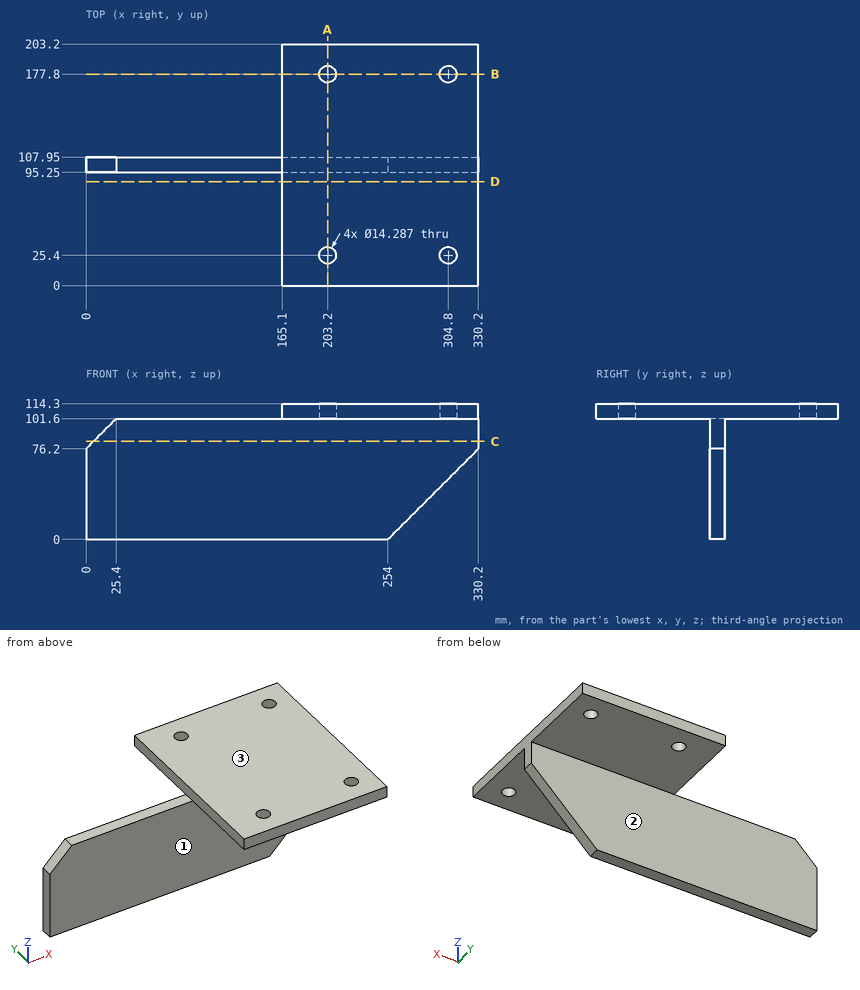
Print and shaded views of the part. All mm, measured from the part's lowest x, y and z. A direction names the side the tool comes from. Coordinates: 2 decimals unless noted, no trailing zeros. Loops run counter-clockwise (first coordinate to the right, second up) from the corner with the lowest first, then second, coordinate; pieces in that order, holes last. Notation, with made-up numbers: (-9.5, 57.25) - (39.5, 57.25) arc R33 cw to (39.5, 94.25) - close; hole circle Ø1 at (-5.5, 66). An arc over 180 degrees is marked (long way). Write item = value, one per line. Start each with the question number.
Item 1: Cut at C-C, the plane z = 82.5. Give the cut face in (x, y).
Item 2: Cut at A-A, the plane x = 203.2. Give the cut face in (y, z).
Item 3: Wall check: L1, parallel to X at y = 177, z = 104; L2, parallel to Y at x = 304.8, z = 107.75; L3, parallel to Y at x = 136.5, z = 57.5. Give the ranges that are in metal, low to high. Write a range as from..to.
Item 4: Flat gauge pins, fed straight in: pin 1 Ø23 at (x, y) = (304.8, 25.4) entering from +Z; pin 2 Ø14 at (x, y) = (95.5, 101) entering from +Z; pin 3 Ø4 at (y, z) = (103, 106) entering from -X; pin 4 Ø2 at (x, z) = (57, 36) entering from +Y. Where does each tip first touch, or does it go through?
Item 5: Cut at D-D, the plane y = 87.5. Give the cut face in (x, z).
Item 6: 3-axis set-ups, long thin cutter, end or side, ignore diameter. For the marked faces 1, 2 and 3: which of +Z, -Z, +X, -X, +Y, -Y reach the whole face in a straight line?
Item 7: Cut at B-B, the plane y = 177.8. Give the cut face in (x, z), and give its area (3 significant figures).
The answers:
q1.outline = (6.3, 95.25) - (330.2, 95.25) - (330.2, 107.95) - (6.3, 107.95) - close
q2.outline = (0, 101.6) - (18.26, 101.6) - (18.26, 114.3) - (0, 114.3) - close; (32.54, 101.6) - (95.25, 101.6) - (95.25, 0) - (107.95, 0) - (107.95, 101.6) - (170.66, 101.6) - (170.66, 114.3) - (32.54, 114.3) - close; (184.94, 101.6) - (203.2, 101.6) - (203.2, 114.3) - (184.94, 114.3) - close
q3.L1 = 165.1..196.1, 210.3..297.7, 311.9..330.2
q3.L2 = 0..18.26, 32.54..170.66, 184.94..203.2
q3.L3 = 95.25..107.95
q4.pin_1 = 114.3
q4.pin_2 = 101.6
q4.pin_3 = 165.1
q4.pin_4 = 107.95
q5.outline = (165.1, 101.6) - (330.2, 101.6) - (330.2, 114.3) - (165.1, 114.3) - close
q6.face_1 = -Z, +X, -X, -Y
q6.face_2 = -Z, +X, -X, +Y
q6.face_3 = +Z, +X, -X, +Y, -Y
q7.outline = (165.1, 101.6) - (196.06, 101.6) - (196.06, 114.3) - (165.1, 114.3) - close; (210.34, 101.6) - (297.66, 101.6) - (297.66, 114.3) - (210.34, 114.3) - close; (311.94, 101.6) - (330.2, 101.6) - (330.2, 114.3) - (311.94, 114.3) - close
q7.area = 1,730 mm2
